Part model, mm, in its own coordinate system. A direction names the side the tool comes from. Coordinates: 2 decimals unless noted, no trailing zeros. Loops run counter-clockwise (first coordinate to the right, second up) from the corner with the lowest first, then second, coordinate; pieces in that order, holes last. Notation, with made-up numbers: M -19,10 L -7,10 A16 ccw -7,14 Z; hole C -35.5,18 d4. An arc over 180 degrees is marked long. Answer as a JSON object with one key per item and string values. Group by question number.
1. 3-axis set-ups, long thin cutter, end or side, ignore diameter. For faces 4 (the face through (30, 20, 3.5)), 5 (the face through (30, 20, -3.5)), 6 (the face through (20.496, -1.014, -0.425)), 7 (the face through (2.177, -1.014, 23.852)), 8 (the face through (2.5, 6, 26)): which of +Z, -Z, +X, -X, +Y, -Y reach the whole face in a straight line?
2. Saw through at B-B on x = 12. Write the cut outline in (y, z), then the cut area to 3 significant figures.
3. Mould opens along Y. For faces 1 (the face through (30, 23, 0)), 2 (the face through (27, 15, 0)), 3 (the face through (19.811, 4.902, -19.073)) say: released by +Y, released by -Y, zero draft, split by the parting line, or undercut.
4. Drill centre lines: L1, parallel to Y at x = 26, z = -2; L2, parallel to Y at x = 24, z = 1; L3, parallel to X at y = 8.25, z = 2.5. Where is each one in solid material? Low to high.
5. Saw through at C-C on x = 31. Write the cut outline in (y, z).
6. Drop flat-ended pins along their axis: pin 1 Ø2.5 at (y, z) = (20.5, 0.5) entering from -X; pin 2 Ø19 at (x, z) = (11, -2) entering from +Y; pin 3 Ø5 at (y, z) = (6, 20) entering from +X; pin 4 Ø1.5 at (x, y) = (24.5, 16) entering from -Z (1 decimal). Give the stop position or say it passes through.
7. Saw through at A-A on y = 8.25. Write the cut outline in (x, z), then the cut area to 3 significant figures.
8. Saw through at D-D on z = 22.5. Write the cut outline in (x, y), then the cut area to 3 significant figures.
from build123d import *

# Parameters (mm, degrees)
BOSS_EXTRUDE1_DEPTH = 12
BOSS_EXTRUDE2_START = -2
BOSS_EXTRUDE2_DEPTH = 2
SKETCH4_W           = 6
SKETCH4_H           = 4
BOSS_EXTRUDE3_DEPTH = 20
SKETCH5_W           = 10
SKETCH5_H           = 7
BOSS_EXTRUDE4_DEPTH = 5


with BuildPart() as part:
    # Sketch1 → Boss-Extrude1 (new body)
    with BuildSketch(Plane(origin=(0, 0, 0), x_dir=(1, 0, 0), z_dir=(0, 1, 0))):
        with BuildLine():
            Line((2.5, 27.386127875), (2.5, 25.377155081))
            ThreePointArc((2.5, 25.377155081), (25.5, 0), (2.5, -25.377155081))
            Line((2.5, -25.377155081), (2.5, -27.386127875))
            ThreePointArc((2.5, -27.386127875), (27.5, 0), (2.5, 27.386127875))
        make_face()
    extrude(amount=BOSS_EXTRUDE1_DEPTH)

    # Sketch2 → Boss-Extrude2 (add)
    with BuildSketch(Plane(origin=(0, 0, 0), x_dir=(1, 0, 0), z_dir=(0, 1, 0)).offset(BOSS_EXTRUDE2_START)):
        with BuildLine():
            Line((2.5, 27.386127875), (1.863636364, 20.415113507))
            ThreePointArc((1.863636364, 20.415113507), (20.5, 0), (1.863636364, -20.415113507))
            Line((1.863636364, -20.415113507), (2.5, -27.386127875))
            ThreePointArc((2.5, -27.386127875), (27.5, 0), (2.5, 27.386127875))
        make_face()
    extrude(amount=BOSS_EXTRUDE2_DEPTH)

    # Sketch4 → Boss-Extrude3 (add)
    with BuildSketch(Plane(origin=(0, -2, 0), x_dir=(1, 0, 0), z_dir=(0, 1, 0))):
        with Locations((30, 0)):
            Rectangle(SKETCH4_W, SKETCH4_H)
    extrude(amount=BOSS_EXTRUDE3_DEPTH)

    # Sketch5 → Boss-Extrude4 (add)
    with BuildSketch(Plane(origin=(0, 18, 0), x_dir=(1, 0, 0), z_dir=(0, 1, 0))):
        with Locations((30, 0)):
            Rectangle(SKETCH5_W, SKETCH5_H)
    extrude(amount=BOSS_EXTRUDE4_DEPTH)


solid = part.part
Outcome:
{
 "1": {"face 4": "+Z, +X, -X, +Y", "face 5": "-Z, +X, -X, +Y", "face 6": "-X, +Y, -Y", "face 7": "+Z, -X, +Y, -Y", "face 8": "+Z, -Z, -X, +Y"},
 "2": {"outline": "M -2,-24.74 L 12,-24.74 L 12,-22.5 L 0,-22.5 L 0,-16.62 L -2,-16.62 Z; M -2,16.62 L 0,16.62 L 0,22.5 L 12,22.5 L 12,24.74 L -2,24.74 Z", "area": "86.3 mm²"},
 "3": {"face 1": "released by +Y", "face 2": "undercut", "face 3": "zero draft"},
 "4": {"L1": "y = -2 to 12, 18 to 23", "L2": "y = -2 to 0", "L3": "x = 25.38 to 27.39"},
 "5": {"outline": "M -2,-2 L 18,-2 L 18,-3.5 L 23,-3.5 L 23,3.5 L 18,3.5 L 18,2 L -2,2 Z"},
 "6": {"pin 1": "stops at x = 25", "pin 2": "stops at y = 0", "pin 3": "stops at x = 21.21", "pin 4": "passes through"},
 "7": {"outline": "M 2.5,-27.39 A27.5 ccw 27.43,-2 L 33,-2 L 33,2 L 27.43,2 A27.5 ccw 2.5,27.39 L 2.5,25.38 A25.5 cw 2.5,-25.38 Z", "area": "179 mm²"},
 "8": {"outline": "M 2.05,-2 L 15.81,-2 L 15.81,12 L 12,12 L 12,0 L 2.05,0 Z", "area": "73.3 mm²"}
}
